Geometry check sheet. Reference: the model listing, model coordinates, mm. Face numbers are marked on the shaded views. A direction names the side the tool comes from. Round coordinates to 2 decimals unless told otherwise and drop trailing zeros. Order: outer loops, then holes, each group sorted by start corner. A loop starts at its lowest first (then second) coordinate and runs counter-clockwise, first axis right, second up.
(1) Thickness scan on L1, parallel to X at y = 34, z = 37; L2, parallel to Y at x = -64, z = 52; L3, parallel to X at y = 7, z = 35. Record the ranges inside material, lowest first.
(2) Cross-section at D-D on x = -73. Enter the section's corners in (y, z).
(3) Gauge pin test, flat ends, axial feed: P1, Ø8, axis at x = 34.5, z = 34.5, coming from the +Y side; P2, Ø8, axis at y = 21.5, z = 22, coming from the +X side; P3, Ø3, axis at x = -44.5, z = 15.5, coming from the +Y side. Record the tip position at first contact, or that the pin passes through.
(4) Cross-section at B-B on z = 9. Enter the section's corners in (x, y).
(5) Cross-section at A-A on x = 11.5. Enter the section's corners in (y, z).
(6) Set-up check for the marked faces 1 and 2: record each of +Z, -Z, +X, -X, +Y, -Y from which the full face is reachable in a straight line by a thin tool's end or side.
(7) Cross-section at C-C on y = 35.5. Enter the section's corners in (x, z), and give its area (3 significant figures).
from build123d import *

# Parameters (mm, degrees)
EXTRUDE1_DEPTH      = 40
EXTRUDE1_DEPTH_BACK = 78.25
EXTRUDE2_DEPTH      = 31.755
EXTRUDE4_DEPTH      = 51.755
SKETCH7_W           = 50.762718211
SKETCH7_H           = 77.693391575
CUT_EXTRUDE1_DEPTH  = 10
SKETCH8_W           = 180.54307219
SKETCH8_H           = 130.318791492
CUT_EXTRUDE2_DEPTH  = 40
SKETCH9_W           = 213.468812953
SKETCH9_H           = 29.374372581
CUT_EXTRUDE3_DEPTH  = 32.754264805
EXTRUDE5_DEPTH      = 57.75


with BuildPart() as part:
    # Sketch2 → Extrude1 (new body, two sides)
    with BuildSketch(Plane(origin=(0, 0, 0), x_dir=(0, 0, -1), z_dir=(1, 0, 0))) as extrude1_sk:
        Polygon((0, 0), (0, 31.754264805), (-55, 0), align=None)
    extrude(amount=EXTRUDE1_DEPTH)
    extrude(extrude1_sk.sketch, amount=-EXTRUDE1_DEPTH_BACK)

    # Sketch4 → Extrude2 (add, symmetric)
    with BuildSketch(Plane(origin=(-11.6225, 0, -20.130760511), x_dir=(0.866025404, 0, -0.5), z_dir=(0.5, 0, 0.866025404))):
        Polygon((-95.266487846, 0), (-57.423228684, 31.754264805), (-57.423228684, 0), align=None)
    extrude(amount=EXTRUDE2_DEPTH, both=True)

    # Sketch6 → Extrude4 (add, symmetric)
    with BuildSketch(Plane(origin=(-1.270622992, 0, 2.200783579), x_dir=(0.866025404, 0, 0.5), z_dir=(-0.5, 0, 0.866025404))):
        Polygon((34.641016151, 31.754264805), (79.990806139, 0), (34.641016151, 0), align=None)
    extrude(amount=EXTRUDE4_DEPTH, both=True)

    # Sketch7 → Cut-Extrude1 (cut)
    with BuildSketch(Plane(origin=(-34.088334257, 46.909587917, 19.68090896), x_dir=(-0.830733451, -0.513322613, -0.215364408), z_dir=(-0.556670399, 0.766044443, 0.321393805))):
        with Locations((42.354713251, 21.026293217)):
            Rectangle(SKETCH7_W, SKETCH7_H)
    extrude(amount=CUT_EXTRUDE1_DEPTH, mode=Mode.SUBTRACT)

    # Sketch8 → Cut-Extrude2 (cut)
    with BuildSketch(Plane(origin=(0, 23.815698604, 13.75), x_dir=(-1, 0, 0), z_dir=(0, 0.866025404, 0.5))):
        with Locations((7.268110747, 13.895626923)):
            Rectangle(SKETCH8_W, SKETCH8_H)
    extrude(amount=CUT_EXTRUDE2_DEPTH, mode=Mode.SUBTRACT)

    # Sketch9 → Cut-Extrude3 (cut, through all)
    with BuildSketch(Plane(origin=(0, 0, 0), x_dir=(1, 0, 0), z_dir=(0, 1, 0))):
        with Locations((-3.268792127, 14.685339576)):
            Rectangle(SKETCH9_W, SKETCH9_H)
    extrude(amount=CUT_EXTRUDE3_DEPTH, mode=Mode.SUBTRACT)

    # Sketch1 → Extrude5 (add)
    with BuildSketch(Plane(origin=(0, 0, 0), x_dir=(1, 0, 0), z_dir=(0, 1, 0))):
        with BuildLine():
            Line((40, 0), (-40, 0))
            ThreePointArc((-40, 0), (0, -40), (40, 0))
        make_face()
    extrude(amount=EXTRUDE5_DEPTH)


solid = part.part
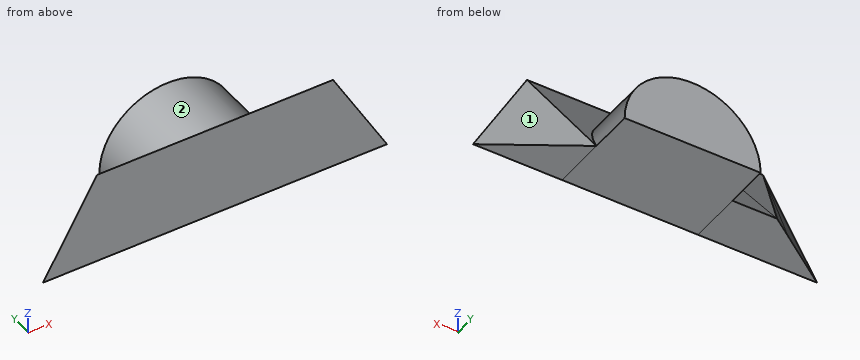
Found:
1. L1: x = -15.2 to 15.2
1. L2: y = 0 to 1.73
1. L3: x = -80.16 to 60.61
2. outline: (0, 0) - (26.89, 0) - (13.96, 30.82) - (0, 55) - close
3. P1: stops at y = 14.15
3. P2: stops at x = 51.2
3. P3: stops at y = 23.67
4. outline: (-104.81, 0) - (87.17, 0) - (43.37, 26.56) - (38.97, 26.56) - (38.97, 57.75) - (-38.97, 57.75) - (-38.97, 26.56) - (-68.26, 26.56) - close
5. outline: (0, 0) - (57.75, 0) - (57.75, 38.31) - (9.64, 38.31) - (0, 55) - close
6. face 1: +Z, +X, +Y
6. face 2: +Z, +Y
7. outline: (-40, 0) - (40, 0) arc R40 ccw to start
7. area: 2,510 mm2
